The listing builds one solid part. Answer for the finished solid, in the listing's coordinates (mm). Give positions to 0.01 mm unless a question says otherwise; leave off trailing zeros. Order: outer loops, then holes, each group sorted by start corner. A loop starts at its lowest first (then second) coordinate and runs counter-clockwise, first axis right, second up.
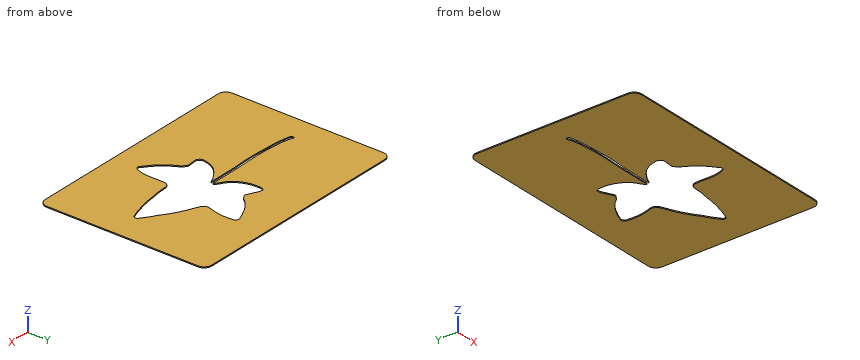
```python
from build123d import *

# Parameters (mm, degrees)
F0_W     = 90.085417
F0_H     = 65
F1_DEPTH = 0.4
F2_R     = 3


with BuildPart() as f1:
    # F0 (on Top) → F1 (new body)
    with BuildSketch(Plane.XY):
        with Locations((-34.513384, 71.062082)):
            Rectangle(F0_W, F0_H)
        with BuildLine():
            ThreePointArc((-69.733061, 72.252296), (-70.037452, 72.9657), (-69.733061, 73.679104))
            ThreePointArc((-69.733061, 73.679104), (-66.277666, 72.662249), (-62.699161, 72.252296))
            ThreePointArc((-62.699161, 72.252296), (-56.899597, 71.827041), (-51.084463, 71.826756))
            ThreePointArc((-51.084463, 71.826756), (-41.736311, 72.036863), (-32.385804, 72.027013))
            ThreePointArc((-32.385804, 72.027013), (-32.447617, 72.318587), (-32.651793, 72.535723))
            ThreePointArc((-32.651793, 72.535723), (-33.37165, 73.170547), (-34.182325, 73.684357))
            ThreePointArc((-34.182325, 73.684357), (-36.052225, 75.011267), (-37.525058, 76.768532))
            ThreePointArc((-37.525058, 76.768532), (-39.105383, 80.56787), (-39.390337, 84.672891))
            ThreePointArc((-39.390337, 84.672891), (-39.30775, 85.296264), (-39.05791, 85.873321))
            ThreePointArc((-39.05791, 85.873321), (-38.593882, 86.426245), (-37.87595, 86.501233))
            ThreePointArc((-37.87595, 86.501233), (-36.667039, 86.0877), (-35.5305, 85.503958))
            ThreePointArc((-35.5305, 85.503958), (-34.511515, 85.040205), (-33.517476, 84.525146))
            ThreePointArc((-33.517476, 84.525146), (-32.714112, 84.219204), (-31.910747, 84.525146))
            ThreePointArc((-31.910747, 84.525146), (-30.891398, 85.144555), (-30.082405, 86.021066))
            ThreePointArc((-30.082405, 86.021066), (-28.817194, 87.387275), (-27.349122, 88.532723))
            ThreePointArc((-27.349122, 88.532723), (-25.759662, 89.611592), (-24.049083, 90.485811))
            ThreePointArc((-24.049083, 90.485811), (-22.169199, 91.371722), (-20.222886, 92.100188))
            ThreePointArc((-20.222886, 92.100188), (-19.418078, 92.135667), (-18.750982, 91.684051))
            ThreePointArc((-18.750982, 91.684051), (-18.451897, 90.696025), (-18.398469, 89.665107))
            ThreePointArc((-18.398469, 89.665107), (-18.492328, 85.684673), (-19.423964, 81.813663))
            ThreePointArc((-19.423964, 81.813663), (-19.655131, 81.135512), (-19.808523, 80.435656))
            ThreePointArc((-19.808523, 80.435656), (-19.524158, 79.083881), (-18.526657, 78.128293))
            ThreePointArc((-18.526657, 78.128293), (-16.473627, 77.251073), (-14.404099, 76.41352))
            ThreePointArc((-14.404099, 76.41352), (-10.122537, 74.16568), (-6.154825, 71.401298))
            ThreePointArc((-6.154825, 71.401298), (-3.695329, 69.924312), (-1.429767, 68.164244))
            ThreePointArc((-1.429767, 68.164244), (-0.713523, 67.146137), (-1.429767, 66.12803))
            ThreePointArc((-1.429767, 66.12803), (-3.227955, 65.416387), (-5.084508, 64.874977))
            ThreePointArc((-5.084508, 64.874977), (-9.976943, 63.629856), (-14.978415, 62.943183))
            ThreePointArc((-14.978415, 62.943183), (-17.926019, 62.451714), (-20.911293, 62.317375))
            ThreePointArc((-20.911293, 62.317375), (-22.521594, 61.884738), (-23.443695, 60.495503))
            ThreePointArc((-23.443695, 60.495503), (-23.475992, 57.653382), (-23.443695, 54.811262))
            ThreePointArc((-23.443695, 54.811262), (-23.670886, 51.635211), (-24.755443, 48.641443))
            ThreePointArc((-24.755443, 48.641443), (-25.632093, 47.926504), (-26.668407, 48.380055))
            ThreePointArc((-26.668407, 48.380055), (-27.048379, 48.641443), (-27.378937, 48.963055))
            ThreePointArc((-27.378937, 48.963055), (-31.240313, 52.474908), (-34.11299, 56.832783))
            ThreePointArc((-34.11299, 56.832783), (-35.046077, 58.204971), (-36.411949, 59.14728))
            ThreePointArc((-36.411949, 59.14728), (-37.906014, 59.079419), (-39.394673, 58.935445))
            ThreePointArc((-39.394673, 58.935445), (-41.29149, 59.47788), (-41.672554, 61.413582))
            ThreePointArc((-41.672554, 61.413582), (-40.874342, 64.095279), (-39.394673, 66.469982))
            ThreePointArc((-39.394673, 66.469982), (-36.262975, 69.133012), (-32.618675, 71.035206))
            ThreePointArc((-32.618675, 71.035206), (-35.665717, 71.099965), (-38.712759, 71.035206))
            ThreePointArc((-38.712759, 71.035206), (-41.521297, 71.056807), (-44.329915, 71.061701))
            ThreePointArc((-44.329915, 71.061701), (-48.366856, 70.808622), (-52.411202, 70.743747))
            ThreePointArc((-52.411202, 70.743747), (-56.196688, 70.850198), (-59.977759, 71.061701))
            ThreePointArc((-59.977759, 71.061701), (-63.884718, 71.260632), (-67.755558, 71.826756))
            ThreePointArc((-67.755558, 71.826756), (-68.747937, 72.022667), (-69.733061, 72.252296))
        make_face(mode=Mode.SUBTRACT)
    extrude(amount=F1_DEPTH)

    # F2
    f2_edges = [f1.edges().sort_by_distance(p)[0] for p in [
        (-79.556093, 38.562082, 0.2),
        (-79.556093, 103.562082, 0.2),
        (10.529324, 38.562082, 0.2),
        (10.529324, 103.562082, 0.2),
    ]]
    fillet(f2_edges, radius=F2_R)


solid = f1.part
```
1) Find section B-B (x = -3). Write down the section's boundary in (y, z).
Geometry says:
outline: (38.56, 0) - (65.5, 0) - (65.5, 0.4) - (38.56, 0.4) - close; (69.43, 0) - (103.56, 0) - (103.56, 0.4) - (69.43, 0.4) - close
2) Straight lines are drawn through the part: probe 1 along Y at (x, z) = (-51, 0.1); probe 2 along X at (y, z) = (83, 0.1); probe 3 along X at (y, z) = (60, 0.25). For each, find the intervals that lie inside material, in ascending order.
Geometry says:
probe 1: y = 38.56 to 70.74, 71.83 to 103.56
probe 2: x = -79.56 to -39.44, -19.04 to 10.53
probe 3: x = -79.56 to -41.63, -23.45 to 10.53
3) Find section A-A (x = -12.5). Write down the section's boundary in (y, z), then the cut area to 3 significant figures.
Geometry says:
outline: (38.56, 0) - (63.21, 0) - (63.21, 0.4) - (38.56, 0.4) - close; (75.5, 0) - (103.56, 0) - (103.56, 0.4) - (75.5, 0.4) - close
area: 21.1 mm2
